Can you work these out from the drawing? Everything is in mm from the part's minimum corner. A direction names the side the tool comes from. Give positions to 0.01 mm unless a question says otherwise; leave off trailing zeros. Write each loop counter-clockwise with the first axis right and the second up, starting at its lowest first coordinate (ties: lowest second). Pieces come first, ordered by that corner, then holes. Notation, with made-up numbers: (54, 26.25) - (85, 26.25) arc R38 ccw to (85, 65.25) - close; hole circle Ø11 at (13.25, 4). An arc over 180 degrees is marked (long way). Return JSON: item names as keys, results as strings. Group by question number.
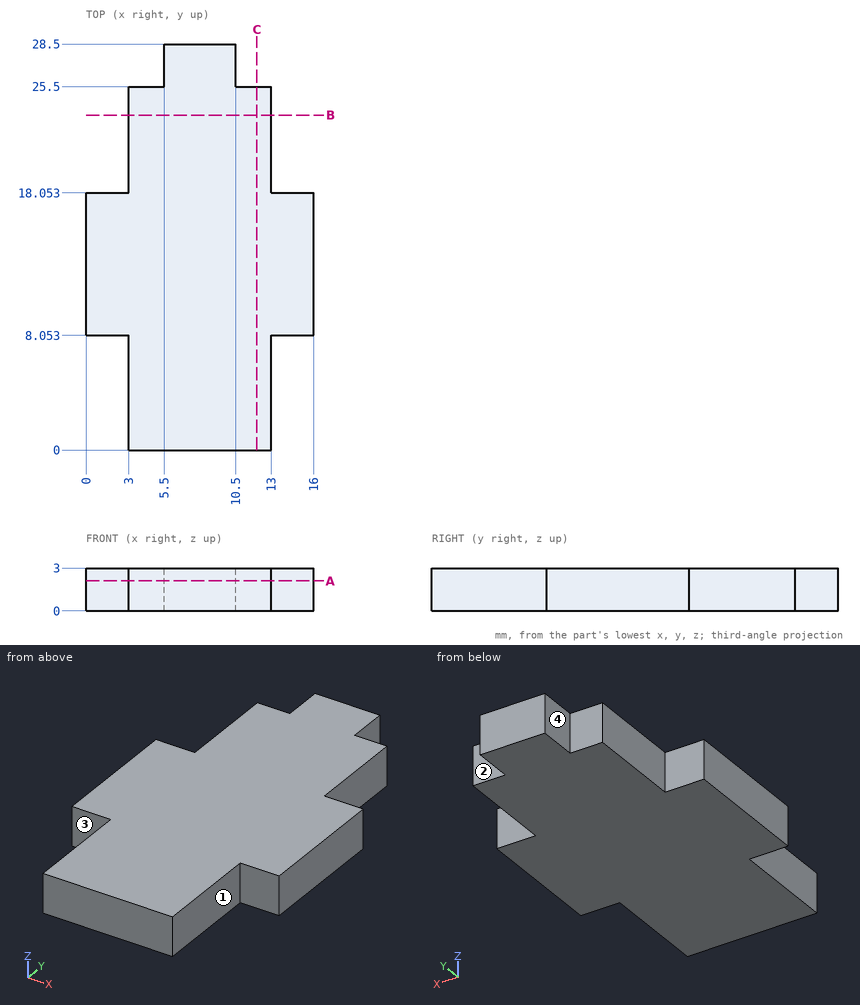
1) I need wall thicknesses on line 1 along X through (y, z) = (26.25, 0.75); line 2 along X through (y, z) = (8, 1.05); line 3 along Y through (x, z) = (5, 0.7). Which ranges of each line are inside material? Lowest first, please.
2) Imagine slicing it at A-A, the plane z = 2.1. Write out the boundary of the cut face in (x, y), and give its area (3 significant figures).
3) Will these pins go through, and if not, where does the flat tip stop? pin 1 Ø1.2 at (x, z) = (4, 2) entering from +Y; pin 2 Ø1.5 at (y, z) = (5, 1) entering from -X; pin 3 Ø0.9 at (x, z) = (14.5, 1) entering from -Y.
4) On a 3-axis mill with a long thin cutter (end or side, diameter ignored), from which of +Z, -Z, +X, -X, +Y, -Y can I reach the whole of each face in a straight line? I mean the marked faces 1, 2, 3 and 4. Say none if no direction works.
5) Imagine slicing it at C-C, the plane x = 12. Write out the boundary of the cut face in (y, z).
6) Imagine slicing it at B-B, the plane y = 23.5. Write out the boundary of the cut face in (x, z).
Resolved:
{
 "1": {"line 1": "5.5 to 10.5", "line 2": "3 to 13", "line 3": "0 to 25.5"},
 "2": {"outline": "(0, 8.05) - (3, 8.05) - (3, 0) - (13, 0) - (13, 8.05) - (16, 8.05) - (16, 18.05) - (13, 18.05) - (13, 25.5) - (10.5, 25.5) - (10.5, 28.5) - (5.5, 28.5) - (5.5, 25.5) - (3, 25.5) - (3, 18.05) - (0, 18.05) - close", "area": "330 mm^2"},
 "3": {"pin 1": "y = 25.5", "pin 2": "x = 3", "pin 3": "y = 8.05"},
 "4": {"face 1": "+Z, -Z, +X, -Y", "face 2": "+Z, -Z, +X, +Y", "face 3": "+Z, -Z, -X, -Y", "face 4": "+Z, -Z, -X, +Y"},
 "5": {"outline": "(0, 0) - (25.5, 0) - (25.5, 3) - (0, 3) - close"},
 "6": {"outline": "(3, 0) - (13, 0) - (13, 3) - (3, 3) - close"}
}
